For this review, take the finished solid that the model builds, in its own axes (mm). Face numbers are marked on the shaded views. A direction names the side the tool comes from. Coordinates: 2 decimals unless noted, no trailing zeros. Order: outer loops, then holes, each group sorted by start corner. A loop starts at its lowest first (then second) coordinate and runs counter-clockwise, first axis right, second up. Notation, with made-up numbers: (85, 16.5) -> (111, 16.5) arc R14 cw to (111, 25.5) -> close; hole circle Ø11 at (87, 1.25). An arc over 180 degrees is marked (long way). Write item = value, one per line. Start each with the question number.
1) Insertion check: pin 1 Ø2 at (y, z) = (-43, 16) entering from +X; pin 2 Ø12.5 at (y, z) = (4.5, 15) entering from -X. Each pin has a flat end and moves straight along its axis. Give the tip position at first contact, or say it passes through.
2) Consider section C-C on x = 63. Give the boundary of the cut face in (y, z).
3) Machinability: for the marked faces 4 and 5, which of the approach directions +Z, -Z, +X, -X, +Y, -Y give a long, thin tool a straight path to every point of the face, cutting with its end or side? Answer none if there is none.
4) Draft analysis for pull direction X (two halves, no side actions). For the marked faces 1, 2 and 3, state which applies: +X half, -X half, draft (parallel to the pull), parting line (faces both ways), or undercut.
5) Consider section B-B on y = 0. Give the boundary of the cut face in (x, z).
6) Consider section A-A on x = 0. Give the boundary of the cut face in (y, z), and give its area (3 significant figures).
7) Consider section D-D on y = 87. Give the boundary of the cut face in (x, z), and give its area (3 significant figures).
8) Wall thickness on probe 1 along X at (y, z) = (63, 6.5); probe 2 along Y at (x, z) = (-63, 17); probe 3 along Y at (x, z) = (42, 19.75): over which ranges is each line inside the solid? List them lowest first. Write a range as [from, to].
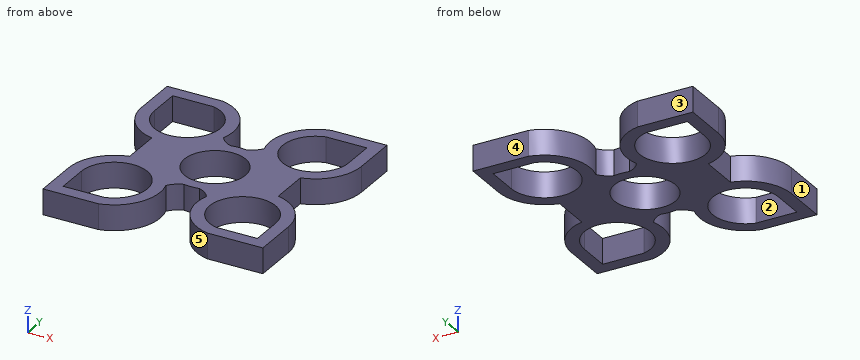
from build123d import *

# Parameters (mm, degrees)
SKETCH1_R           = 30
BOSS_EXTRUDE1_DEPTH = 25


with BuildPart() as part:
    # Sketch1 → Boss-Extrude1 (new body)
    with BuildSketch(Plane.XY):
        with BuildLine():
            ThreePointArc((73, 19.125178063), (98.178118199, 34.937569599), (108, 63))
            Line((108, 63), (108, 107))
            Line((108, 107), (53.566018868, 107))
            ThreePointArc((53.566018868, 107), (24.177408949, 85.755360338), (20, 49.733500839))
            ThreePointArc((20, 49.733500839), (14.637539739, 43.980472393), (7.703238546, 40.26984127))
            ThreePointArc((7.703238546, 40.26984127), (0, 41), (-7.703238546, 40.26984127))
            ThreePointArc((-7.703238546, 40.26984127), (-14.637539739, 43.980472393), (-20, 49.733500839))
            ThreePointArc((-20, 49.733500839), (-24.177408949, 85.755360338), (-53.566018868, 107))
            Line((-53.566018868, 107), (-108, 107))
            Line((-108, 107), (-108, 63))
            ThreePointArc((-108, 63), (-98.178118199, 34.937569599), (-73, 19.125178063))
            Line((-73, 19.125178063), (-73, -19.125178063))
            ThreePointArc((-73, -19.125178063), (-98.178118199, -34.937569599), (-108, -63))
            Line((-108, -63), (-108, -107))
            Line((-108, -107), (-53.566018868, -107))
            ThreePointArc((-53.566018868, -107), (-24.177408949, -85.755360338), (-20, -49.733500839))
            ThreePointArc((-20, -49.733500839), (-14.637539739, -43.980472393), (-7.703238546, -40.26984127))
            ThreePointArc((-7.703238546, -40.26984127), (0, -41), (7.703238546, -40.26984127))
            ThreePointArc((7.703238546, -40.26984127), (14.637539739, -43.980472393), (20, -49.733500839))
            ThreePointArc((20, -49.733500839), (24.177408949, -85.755360338), (53.566018868, -107))
            Line((53.566018868, -107), (108, -107))
            Line((108, -107), (108, -63))
            ThreePointArc((108, -63), (98.178118199, -34.937569599), (73, -19.125178063))
            Line((73, -19.125178063), (73, 19.125178063))
        make_face()
        with BuildLine():
            Line((95.4, -63), (95.4, -94.4))
            Line((95.4, -94.4), (55.012509781, -94.4))
            ThreePointArc((55.012509781, -94.4), (43.113254202, -37.421154413), (95.4, -63))
        make_face(mode=Mode.SUBTRACT)
        with BuildLine():
            ThreePointArc((-55.012509781, 94.4), (-43.113254202, 37.421154413), (-95.4, 63))
            Line((-95.4, 63), (-95.4, 65.547547841))
            Line((-95.4, 65.547547841), (-95.4, 94.4))
            Line((-95.4, 94.4), (-55.012509781, 94.4))
        make_face(mode=Mode.SUBTRACT)
        Circle(SKETCH1_R, mode=Mode.SUBTRACT)
        with BuildLine():
            Line((55.012509781, 94.4), (95.4, 94.4))
            Line((95.4, 94.4), (95.4, 65.547547841))
            Line((95.4, 65.547547841), (95.4, 63))
            ThreePointArc((95.4, 63), (43.113254202, 37.421154413), (55.012509781, 94.4))
        make_face(mode=Mode.SUBTRACT)
        with BuildLine():
            Line((-95.4, -94.4), (-95.4, -63))
            ThreePointArc((-95.4, -63), (-43.113254202, -37.421154413), (-55.012509781, -94.4))
            Line((-55.012509781, -94.4), (-95.4, -94.4))
        make_face(mode=Mode.SUBTRACT)
    extrude(amount=BOSS_EXTRUDE1_DEPTH)


solid = part.part
Answer sheet:
q1.pin_1 = 103.79
q1.pin_2 = -73
q2.outline = (-107, 0) -> (-94.4, 0) -> (-94.4, 25) -> (-107, 25) -> close; (-30.6, 0) -> (30.6, 0) -> (30.6, 25) -> (-30.6, 25) -> close; (94.4, 0) -> (107, 0) -> (107, 25) -> (94.4, 25) -> close
q3.face_4 = +Z, -Z, +X, -X, +Y
q3.face_5 = +Z, -Z
q4.face_1 = -X half
q4.face_2 = undercut
q4.face_3 = draft
q5.outline = (-73, 0) -> (-30, 0) -> (-30, 25) -> (-73, 25) -> close; (30, 0) -> (73, 0) -> (73, 25) -> (30, 25) -> close
q6.outline = (-41, 0) -> (-30, 0) -> (-30, 25) -> (-41, 25) -> close; (30, 0) -> (41, 0) -> (41, 25) -> (30, 25) -> close
q6.area = 550 mm2
q7.outline = (-108, 0) -> (-95.4, 0) -> (-95.4, 25) -> (-108, 25) -> close; (-41.23, 0) -> (-24.93, 0) -> (-24.93, 25) -> (-41.23, 25) -> close; (24.93, 0) -> (41.23, 0) -> (41.23, 25) -> (24.93, 25) -> close; (95.4, 0) -> (108, 0) -> (108, 25) -> (95.4, 25) -> close
q7.area = 1,440 mm2
q8.probe_1 = [-108, -95.4], [-30.6, -18], [18, 30.6], [95.4, 108]
q8.probe_2 = [-107, -94.4], [-30.6, 30.6], [94.4, 107]
q8.probe_3 = [-102.8, -87.67], [-38.33, 38.33], [87.67, 102.8]
